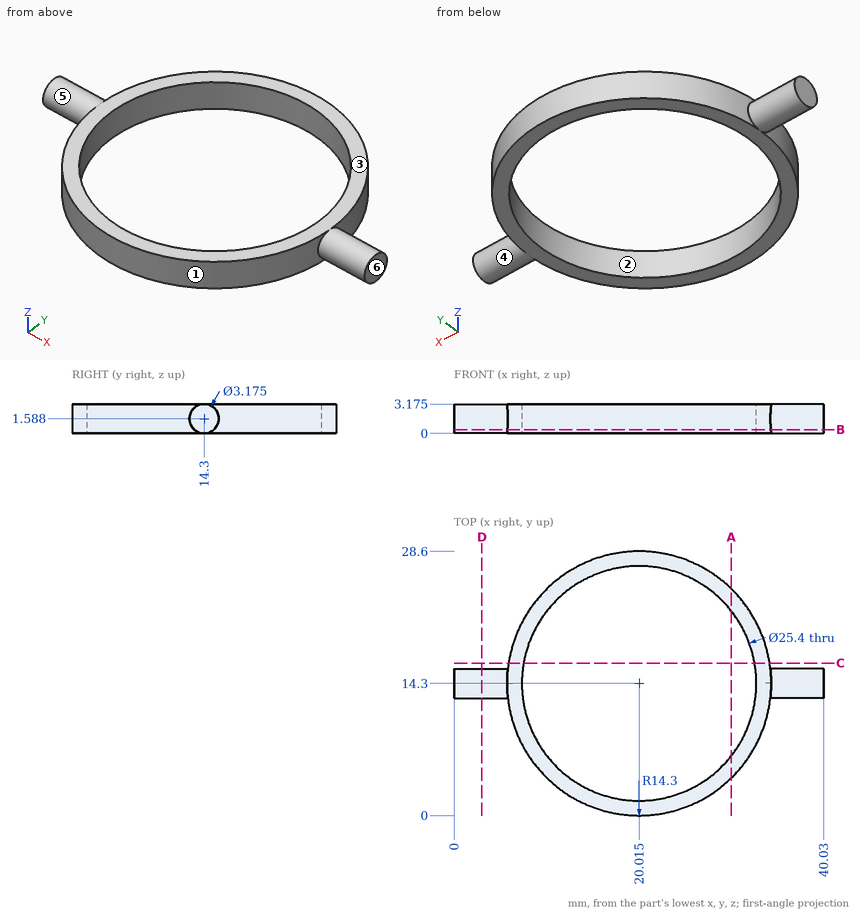
The drawing under review shows one solid part. Ordinate dimensions are in mm from its lowest x, y, z. A direction names the side the tool comes from. Give positions to 0.01 mm unless a question says otherwise; leave off trailing zeros. Order: outer loops, then holes, each group sorted by start corner. A loop starts at its lowest first (then second) coordinate and runs counter-clockwise, first axis right, second up. Notation, with made-up numbers: M 76,9.25 L 85,9.25 A20 cw 85,37.25 Z; hole C -25.5,27 d10. An arc over 180 degrees is marked long. One line per question, with ' | ' between items. Start each with the question number.
Q1. For pin 1 Ø1 at (y, z) = (8.5, 0.5) entering from -X; pin 2 Ø1 at (y, z) = (4.5, 2) entering from +X, all flat-tipped, find the tip position at first contact; note any pin that passes through.
Q2. We need section B-B (z = 0.4). Write out the cut boundary in (x, y) (1 decimal), plus the area to 3 significant figures.
Q3. For L1, parallel to Y at x = 21.5, z = 0.5; L2, parallel to Y at x = 18, z = 1.65; L3, parallel to X at y = 9.75, z = 2.35, list the stretches that pass through material, from the lowest coordinate up. Write a range as [from, to].
Q4. Machinability: for the marked faces 4, 5 and 6, which of the approach directions +Z, -Z, +X, -X, +Y, -Y give a long, thin tool a straight path to every point of the face, cutting with its end or side? Answer none if there is none.
Q5. The part is to be moulded in two halves that separate along X. For the marked faces 1, 2 and 3, say which applies: +X half, -X half, draft (parallel to the pull), parting line (faces both ways), or undercut.
Q6. We need section C-C (y = 16.5). Write out the cut boundary in (x, z) (1 decimal).
Q7. We need section D-D (x = 3). Write out the cut boundary in (y, z) (1 decimal).
Q8. We need section A-A (x = 30). Write out the cut boundary in (y, z) (1 decimal).
Returned:
1) pin 1: x = 6.73 | pin 2: x = 30.88
2) outline: M 0,13.2 L 5.8,13.2 A14.3 ccw 34.3,13.2 L 40,13.2 L 40,15.4 L 34.3,15.4 A14.3 ccw 5.8,15.4 L 0,15.4 Z; hole C 20,14.3 d25.4 | area: 160 mm2
3) L1: [0.08, 1.69], [26.91, 28.52] | L2: [0.14, 1.76], [26.84, 28.46] | L3: [6.46, 8.16], [31.87, 33.57]
4) face 4: +X | face 5: -X | face 6: +Z, -Z, +X, +Y, -Y
5) face 1: parting line | face 2: undercut | face 3: draft
6) outline: M 5.9,0 L 7.5,0 L 7.5,3.2 L 5.9,3.2 Z; M 32.5,0 L 34.1,0 L 34.1,3.2 L 32.5,3.2 Z
7) outline: C 14.3,1.6 d3.2
8) outline: M 4.1,0 L 6.5,0 L 6.5,3.2 L 4.1,3.2 Z; M 22.1,0 L 24.5,0 L 24.5,3.2 L 22.1,3.2 Z
